Check sheet for the modelled part. Datum: model origin and axes. Units: mm. Face numbers are marked on the shaded views. A direction names the side the tool comes from. Round coordinates to 2 decimals unless told otherwise and drop trailing zeros. Write each loop counter-clockwise with the first axis right and the second up, starting at its lowest first coordinate (ties: lowest second). Pieces come first, ordered by that corner, then holes. Notation, with made-up numbers: M 64,68 L 72,68 A34 ccw 72,106 Z; hole C 19.5,7 d2. An arc over 180 degrees is marked long. Put each result on its own line as item: value.
```python
from build123d import *

# Parameters (mm, degrees)
F0_R     = 8.5
F1_DEPTH = 2
F2_W     = 22
F2_H     = 71.162369
F3_DEPTH = 5


with BuildPart() as f1:
    # F0 (on Front) → F1 (new body)
    with BuildSketch(Plane.XZ):
        with BuildLine():
            Line((26.236077, 16.621207), (-19.205651, 16.621207))
            ThreePointArc((-19.205651, 16.621207), (-34.786835, 1.040022), (-19.205651, -14.541162))
            Line((-19.205651, -14.541162), (26.236077, -14.541162))
            Line((26.236077, -14.541162), (26.236077, 16.621207))
        make_face()
        with Locations((-19.205651, 1.040022)):
            Circle(F0_R, mode=Mode.SUBTRACT)
    extrude(amount=F1_DEPTH)

    # F2 (on face) → F3 (join)
    with BuildSketch(Plane.YZ.offset(26.236077)):
        with Locations((-1, 1.040022)):
            Rectangle(F2_W, F2_H)
    extrude(amount=F3_DEPTH)


solid = f1.part
```
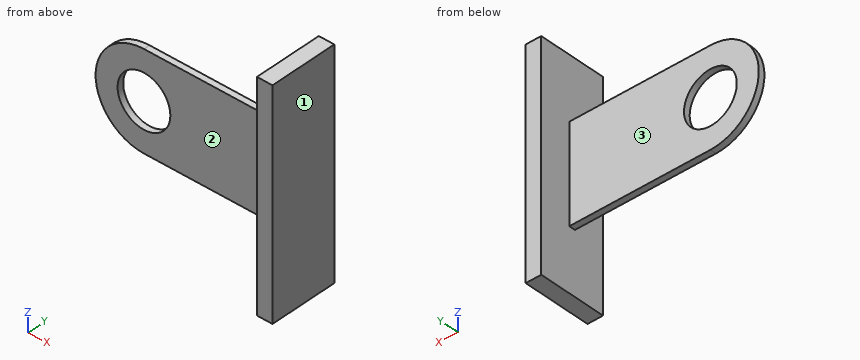
1. Depth check by flat-ended pin: pin 1 Ø12 at (y, z) = (2.5, -17.5) entering from -X; pin 2 Ø10 at (x, z) = (-18.5, 10.5) entering from -Y; pin 3 Ø6.5 at (y, z) = (2.5, -11.5) entering from -X. Enter the tip coordinate at first touch or a pass-through.
Computed values:
pin 1: stops at x = -27.66
pin 2: stops at y = -2
pin 3: stops at x = -30.75
2. Cross-section at D-D (z = 13). Enter the section's corners in (x, y).
Computed values:
outline: M -29.19,-2 L 26.24,-2 L 26.24,-12 L 31.24,-12 L 31.24,10 L 26.24,10 L 26.24,0 L -29.19,0 Z
3. Cross-section at A-A (z = -1). Enter the section's corners in (x, y), then the cut area to 3 significant figures.
Computed values:
outline: M -34.65,-2 L -27.46,-2 L -27.46,0 L -34.65,0 Z; M -10.95,-2 L 26.24,-2 L 26.24,-12 L 31.24,-12 L 31.24,10 L 26.24,10 L 26.24,0 L -10.95,0 Z
area: 199 mm2
4. Scan lines: probe 1 along X at (y, z) = (-5, 24); probe 2 along Y at (x, z) = (-5, -8.5); probe 3 along Z at (x, y) = (-26, -0.25). Record each from-to range of solid material in increasing order.
Computed values:
probe 1: x = 26.24 to 31.24
probe 2: y = -2 to 0
probe 3: z = -12.98 to -4.07, 6.15 to 15.06
5. Cross-section at C-C (y = 7.25). Enter the section's corners in (x, z), then the cut area to 3 significant figures.
Computed values:
outline: M 26.24,-34.54 L 31.24,-34.54 L 31.24,36.62 L 26.24,36.62 Z
area: 356 mm2
6. Cross-section at B-B (x = -24). Enter the section's corners in (y, z).
Computed values:
outline: M -2,-13.79 L 0,-13.79 L 0,-5.98 L -2,-5.98 Z; M -2,8.06 L 0,8.06 L 0,15.87 L -2,15.87 Z
7. Access from +Z, -Z, +X, -X, +Y, -Y to the whole of each face (thin tool, end or side, straight path). Record for the marked faces 1, 2 and 3.
Computed values:
face 1: +Z, -Z, +X, +Y, -Y
face 2: +Z, -Z, -X, -Y
face 3: +Z, -Z, -X, +Y
